Source: three-view drawing plus pictorial views. Frame: mm from the lowest corner of the part. A direction names the side the tool comes from. Coordinates: 2 decimals unless noted, no trailing zeros. Order: outer loops, then holes, each group sorted by start corner. A loop starts at its lowest first (then second) coordinate and runs counter-clockwise, first axis right, second up. Notation, with made-up numbers: M 24,38.25 L 33,38.25 A11 ccw 33,47.25 Z; hole C 56,-3.5 d6. An arc over 180 degrees is marked long. One line per question, with ' | ' between items.
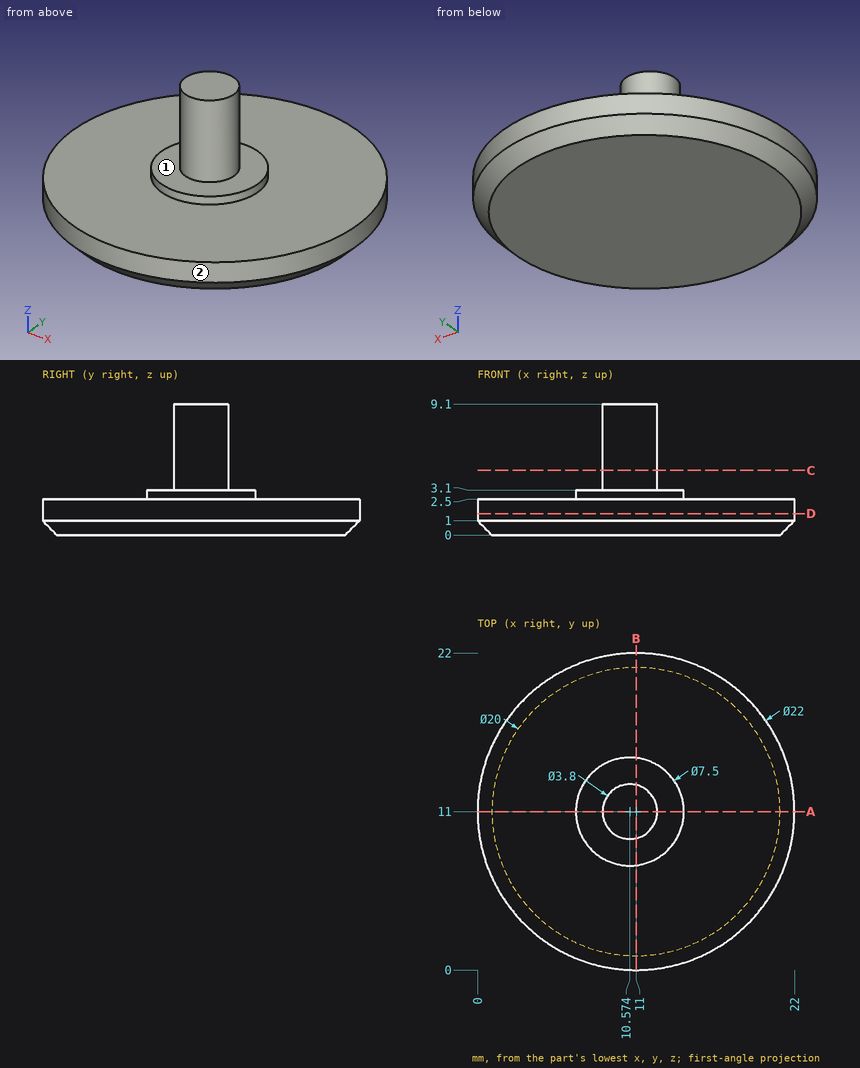
1. Section C-C, the plane z = 4.5. Output: boundary loops of the cut face in (x, y).
Response values:
outline: C 10.57,11 d3.8
2. Material intervals for line 1 (Z direction, x = 17.75, y = 5.5); line 2 (Z direction, x = 9, y = 9.75); line 3 (X direction, y = 5, z = 2), sorted ascending. Write a range as [from, to].
Response values:
line 1: z = [0, 2.5] | line 2: z = [0, 3.1] | line 3: x = [1.78, 20.22]
3. Access query for the marked faces 1 and 2. Directions: +Z, -Z, +X, -X, +Y, -Y. A direction counts if a zero-diameter tool reaches every point of the face in a straight line with its end or side. Return the directions, or none.
Response values:
face 1: +Z | face 2: +Z, -Z
4. Section D-D, the plane z = 1.5. Output: boundary loops of the cut face in (x, y).
Response values:
outline: C 11,11 d22
5. Section A-A, the plane y = 11. Output: boundary loops of the cut face in (x, z).
Response values:
outline: M 0,1 L 1,0 L 21,0 L 22,1 L 22,2.5 L 14.32,2.5 L 14.32,3.1 L 12.47,3.1 L 12.47,9.1 L 8.67,9.1 L 8.67,3.1 L 6.82,3.1 L 6.82,2.5 L 0,2.5 Z
6. Section B-B, the plane x = 11. Output: boundary loops of the cut face in (y, z), and give its area (3 significant figures).
Response values:
outline: M 0,1 L 1,0 L 21,0 L 22,1 L 22,2.5 L 14.73,2.5 L 14.73,3.1 L 12.85,3.1 L 12.85,9.1 L 9.15,9.1 L 9.15,3.1 L 7.27,3.1 L 7.27,2.5 L 0,2.5 Z | area: 80.7 mm^2
7. Pin query (flat end, axial travel): P1, Ø3, axis at x = 7, y = 3.5, coming from the +Z side; P2, Ø1.5, axis at y = 13, z = 6.5, coming from the -X side; P3, Ø12, axis at x = 6, y = 4, coming from the +Z side. Return the tip coordinate at first contact, or that it passes through.
Response values:
P1: stops at z = 2.5 | P2: stops at x = 9.14 | P3: stops at z = 3.1
